```python
from build123d import *

# Parameters (mm, degrees)
BOSS_EXTRUDE1_DEPTH = 10
SKETCH2_R           = 2.5
SKETCH2_W           = 10
SKETCH2_H           = 10
SKETCH2_W_2         = 20
CUT_EXTRUDE1_DEPTH  = 202.804360706
SKETCH4_R           = 2
CUT_EXTRUDE2_DEPTH  = 202.804360706
SKETCH5_W           = 10
SKETCH5_H           = 10
SKETCH5_H_2         = 20
CUT_EXTRUDE3_DEPTH  = 202.804360706


with BuildPart() as part:
    # Sketch3 → Boss-Extrude1 (new body)
    with BuildSketch(Plane(origin=(0, 0, 0), x_dir=(1, 0, 0), z_dir=(0, 1, 0))):
        with BuildLine():
            Line((-100, -75), (100, -75))
            Line((100, -75), (100, 75))
            ThreePointArc((100, 75), (0, 175), (-100, 75))
            Line((-100, 75), (-100, -75))
        make_face()
    extrude(amount=BOSS_EXTRUDE1_DEPTH)

    # Sketch2 → Cut-Extrude1 (cut, through all)
    with BuildSketch(Plane(origin=(0, 10, 0), x_dir=(1, 0, 0), z_dir=(0, 1, 0))):
        with Locations(Location((45, 30, 0), (0, 0, 270))):
            Circle(SKETCH2_R)
        with Locations(Location((45, -50, 0), (0, 0, 270))):
            Circle(SKETCH2_R)
        with Locations(Location((85, -40, 0), (0, 0, 270))):
            Circle(SKETCH2_R)
        with Locations(Location((85, 20, 0), (0, 0, 270))):
            Circle(SKETCH2_R)
        with Locations((35, -50)):
            Rectangle(SKETCH2_W, SKETCH2_H)
        with Locations((55, -50)):
            Rectangle(SKETCH2_W, SKETCH2_H)
        with Locations((80, -50)):
            Rectangle(SKETCH2_W_2, SKETCH2_H)
        with Locations((85, -30)):
            Rectangle(SKETCH2_W, SKETCH2_H)
        with Locations((85, -10)):
            Rectangle(SKETCH2_W, SKETCH2_H)
        with Locations((85, 10)):
            Rectangle(SKETCH2_W, SKETCH2_H)
        with Locations((80, 30)):
            Rectangle(SKETCH2_W_2, SKETCH2_H)
        with Locations((55, 30)):
            Rectangle(SKETCH2_W, SKETCH2_H)
        with Locations((35, 30)):
            Rectangle(SKETCH2_W, SKETCH2_H)
    cut_extrude1 = extrude(amount=-CUT_EXTRUDE1_DEPTH, mode=Mode.SUBTRACT)

    # Mirror1: Cut-Extrude1 across plane
    add(cut_extrude1.mirror(Plane(origin=(0, 0, 0), x_dir=(0, 0, 1), z_dir=(1, 0, 0))), mode=Mode.SUBTRACT)

    # Sketch4 → Cut-Extrude2 (cut, through all)
    with BuildSketch(Plane(origin=(0, 10, 0), x_dir=(1, 0, 0), z_dir=(0, 1, 0))):
        with Locations(Location((55, 125, 0), (0, 0, 270))):
            Circle(SKETCH4_R)
        with Locations(Location((55, 85, 0), (0, 0, 270))):
            Circle(SKETCH4_R)
        with Locations(Location((-55, 125, 0), (0, 0, 270))):
            Circle(SKETCH4_R)
        with Locations(Location((-55, 85, 0), (0, 0, 270))):
            Circle(SKETCH4_R)
        with BuildLine():
            Line((-5, 155), (5, 155))
            ThreePointArc((5, 155), (19.142135624, 149.142135624), (25, 135))
            Line((25, 135), (25, 75))
            ThreePointArc((25, 75), (19.142135624, 60.857864376), (5, 55))
            Line((5, 55), (-5, 55))
            ThreePointArc((-5, 55), (-19.142135624, 60.857864376), (-25, 75))
            Line((-25, 75), (-25, 135))
            ThreePointArc((-25, 135), (-19.142135624, 149.142135624), (-5, 155))
        make_face()
    extrude(amount=-CUT_EXTRUDE2_DEPTH, mode=Mode.SUBTRACT)

    # Sketch5 → Cut-Extrude3 (cut, symmetric)
    with BuildSketch(Plane(origin=(0, 10, 0), x_dir=(1, 0, 0), z_dir=(0, 1, 0))):
        with Locations((80, 50)):
            Rectangle(SKETCH5_W, SKETCH5_H)
        with Locations((60, 50)):
            Rectangle(SKETCH5_W, SKETCH5_H)
        with Locations((40, 50)):
            Rectangle(SKETCH5_W, SKETCH5_H)
        with Locations((5, -10)):
            Rectangle(SKETCH5_W, SKETCH5_H_2)
        with Locations((40, -70)):
            Rectangle(SKETCH5_W, SKETCH5_H)
        with Locations((60, -70)):
            Rectangle(SKETCH5_W, SKETCH5_H)
        with Locations((80, -70)):
            Rectangle(SKETCH5_W, SKETCH5_H)
    cut_extrude3 = extrude(amount=CUT_EXTRUDE3_DEPTH, both=True, mode=Mode.SUBTRACT)

    # Mirror2: Cut-Extrude3 across plane
    add(cut_extrude3.mirror(Plane(origin=(0, 0, 0), x_dir=(0, 0, 1), z_dir=(1, 0, 0))), mode=Mode.SUBTRACT)


solid = part.part
```
Geometry check sheet. Reference: the model listing, model coordinates, mm. A direction names the side the tool comes from. Round coordinates to 2 decimals unless told otherwise and drop trailing zeros. Loops run counter-clockwise (first coordinate to the right, second up) from the corner with the lowest first, then second, coordinate; pieces in that order, holes last. Notation, with made-up numbers: (43, 63.5) - (63, 63.5) arc R25 ccw to (63, 78.5) - close; hole circle Ø10 at (25.25, -23). An arc over 180 degrees is marked (long way). Use a Markdown table: item, result.
Q1. Go/stop test with flat-tipped pins: P1, Ø3, axis at x = -85.5, y = 5, coming from the -Z side; P2, Ø1.5, axis at x = 31.5, z = 49, coming from the -Y side; P3, Ø3, axis at x = 78, y = 7, coming from the +Z side; P4, Ø2, axis at x = -68, y = 7.5, coming from the -Z side. Record where each tip stops, or that it passes through.
Solutions:
| item | result |
|---|---|
| P1 | stops at z = -129.26 |
| P2 | passes through |
| P3 | stops at z = 65 |
| P4 | stops at z = -149.24 |
Q2. Access from +Z, -Z, +X, -X, +Y, -Y to the whole of each face (thin tool, end or side, straight path). Record for faces 1 (the flat face through (60, 5, 65)), 2 (the flat face through (80, 5, 30)).
Solutions:
| item | result |
|---|---|
| face 1 | +Z, +Y, -Y |
| face 2 | +Y, -Y |
Q3. Cross-section at A-A on z = -103. Record the cut outline in (x, y), plus the area to 3 significant figures.
Solutions:
| item | result |
|---|---|
| outline | (-96, 0) - (-25, 0) - (-25, 10) - (-96, 10) - close; (25, 0) - (96, 0) - (96, 10) - (25, 10) - close |
| area | 1,420 mm2 |
Q4. Material ranges on line 1 (X direction, y = 4.75, z = -20); line 2 (Z direction, x = -39, y = 9.5); line 3 (X direction, y = 6, z = -85), recorded low to high.
Solutions:
| item | result |
|---|---|
| line 1 | x = -100 to -87.5, -82.5 to 82.5, 87.5 to 100 |
| line 2 | z = -167.08 to -55, -45 to -35, -25 to 45, 55 to 65 |
| line 3 | x = -99.5 to -57, -53 to -25, 25 to 53, 57 to 99.5 |
Q5. Cross-section at C-C on y = 7. State how many separate pieces and enclosed holes the cut face has, plus the area to 3 significant figures.
Solutions:
| item | result |
|---|---|
| separate pieces | 1 |
| enclosed holes | 38 |
| area | 37,000 mm2 |
Q6. Cross-section at D-D on z = -142. Record the cut outline in (x, y) (3 decimals), plus the area to 3 significant figures.
Solutions:
| item | result |
|---|---|
| outline | (-74.236, 0) - (-23.735, 0) - (-23.735, 10) - (-74.236, 10) - close; (23.735, 0) - (74.236, 0) - (74.236, 10) - (23.735, 10) - close |
| area | 1,010 mm2 |
Q7. Draft check along Z on faces 3 (the flat face through (0, 5, -55)), 4 (the flat face through (50, 5, 75)), 5 (the flat face through (-100, 5, -1)). Enter one of: released by +Z, released by -Z, zero draft, split by the parting line, or undercut.
Solutions:
| item | result |
|---|---|
| face 3 | undercut |
| face 4 | released by +Z |
| face 5 | zero draft |
Q8. Cross-section at B-B on z = -9.5. Record the cut outline in (x, y), plus the area to 3 significant figures.
Solutions:
| item | result |
|---|---|
| outline | (-100, 0) - (-90, 0) - (-90, 10) - (-100, 10) - close; (-80, 0) - (80, 0) - (80, 10) - (-80, 10) - close; (90, 0) - (100, 0) - (100, 10) - (90, 10) - close |
| area | 1,800 mm2 |
